CAD build for the part. Positions are in the model's coordinates, mm. Face numbers are marked on the shaded views. A direction names the side the tool comes from. Coordinates: 2 decimals unless noted, no trailing zeros. Write each loop counter-clockwise with the first axis right and the second up, starting at its lowest first coordinate (ties: lowest second). Pieces come first, ordered by that corner, then holes. Notation, with made-up numbers: (-40, 15) -> (-22, 15) arc R24 ccw to (-22, 38) -> close; hole circle Ø5 at (40.5, -30.5). An arc over 180 degrees is marked (long way). Answer as CSV lines item,"result".
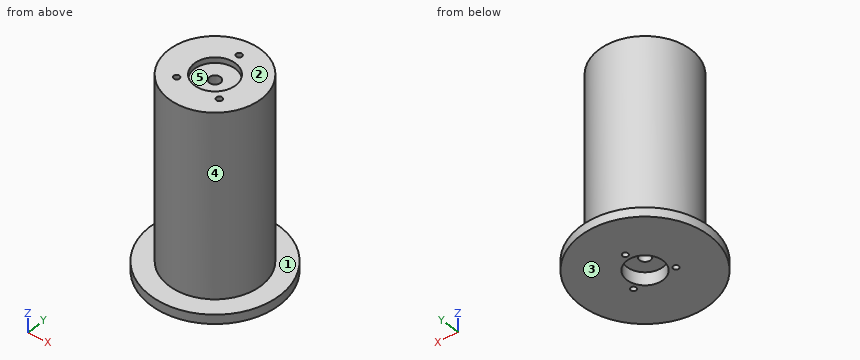
```python
from build123d import *

# Parameters (mm, degrees)
SKETCH_1_R          = 25
EXTRUDE_1_DEPTH     = 100
SKETCH_2_R          = 35
EXTRUDE_2_DEPTH     = 5
SKETCH_4_R          = 9.8
CUT_EXTRUDE_1_DEPTH = 7
SKETCH_5_R          = 3
CUT_EXTRUDE_2_DEPTH = 106
SKETCH_6_R          = 1.5
CUT_EXTRUDE_3_DEPTH = 10
SKETCH_7_R          = 11.15
CUT_EXTRUDE_4_DEPTH = 3
SKETCH_8_R          = 1.55
CUT_EXTRUDE_5_DEPTH = 10


with BuildPart() as part:
    # Эскиз1 → Бобышка-Вытянуть1 (new body)
    with BuildSketch(Plane.XY):
        Circle(SKETCH_1_R)
    extrude(amount=EXTRUDE_1_DEPTH)

    # Эскиз2 → Бобышка-Вытянуть2 (add)
    with BuildSketch(Plane(origin=(0, 0, 0), x_dir=(-1, 0, 0), z_dir=(0, 0, -1))):
        Circle(SKETCH_2_R)
    extrude(amount=EXTRUDE_2_DEPTH)

    # Эскиз4 → Вырез-Вытянуть1 (cut)
    with BuildSketch(Plane(origin=(0, 0, -5), x_dir=(-1, 0, 0), z_dir=(0, 0, -1))):
        Circle(SKETCH_4_R)
    extrude(amount=-CUT_EXTRUDE_1_DEPTH, mode=Mode.SUBTRACT)

    # Эскиз5 → Вырез-Вытянуть2 (cut, through all)
    with BuildSketch(Plane(origin=(0, 0, -5), x_dir=(-1, 0, 0), z_dir=(0, 0, -1))):
        Circle(SKETCH_5_R)
    extrude(amount=-CUT_EXTRUDE_2_DEPTH, mode=Mode.SUBTRACT)

    # Эскиз6 → Вырез-Вытянуть3 (cut)
    with BuildSketch(Plane(origin=(0, 0, -5), x_dir=(-1, 0, 0), z_dir=(0, 0, -1))):
        with Locations((0, 13)):
            Circle(SKETCH_6_R)
        with Locations((11.258330249, -6.5)):
            Circle(SKETCH_6_R)
        with Locations((-11.258330249, -6.5)):
            Circle(SKETCH_6_R)
    extrude(amount=-CUT_EXTRUDE_3_DEPTH, mode=Mode.SUBTRACT)

    # Эскиз7 → Вырез-Вытянуть4 (cut)
    with BuildSketch(Plane.XY.offset(100)):
        Circle(SKETCH_7_R)
    extrude(amount=-CUT_EXTRUDE_4_DEPTH, mode=Mode.SUBTRACT)

    # Эскиз8 → Вырез-Вытянуть5 (cut)
    with BuildSketch(Plane.XY.offset(100)):
        with Locations((0, 16)):
            Circle(SKETCH_8_R)
        with Locations((-11.313708499, -11.313708499)):
            Circle(SKETCH_8_R)
        with Locations((11.313708499, -11.313708499)):
            Circle(SKETCH_8_R)
    extrude(amount=-CUT_EXTRUDE_5_DEPTH, mode=Mode.SUBTRACT)


solid = part.part
```
Item 1: Saw through at D-D on x = 28. Give the cut face in (y, z), and give its area (3 significant figures).
Answer below:
outline,"(-21, -5) -> (21, -5) -> (21, 0) -> (-21, 0) -> close"
area,"210 mm2"
Item 2: Saw through at C-C on y = 13. Give the cut face in (x, z), and give its area (3 significant figures).
Answer below:
outline,"(-32.5, -5) -> (-1.5, -5) -> (-1.5, 5) -> (1.5, 5) -> (1.5, -5) -> (32.5, -5) -> (32.5, 0) -> (21.35, 0) -> (21.35, 100) -> (-21.35, 100) -> (-21.35, 0) -> (-32.5, 0) -> close"
area,"4,570 mm2"
Item 3: Saw through at A-A on x = 0. Give the cut face in (y, z).
Answer below:
outline,"(-35, -5) -> (-9.8, -5) -> (-9.8, 2) -> (-3, 2) -> (-3, 97) -> (-11.15, 97) -> (-11.15, 100) -> (-25, 100) -> (-25, 0) -> (-35, 0) -> close; (3, 2) -> (9.8, 2) -> (9.8, -5) -> (11.5, -5) -> (11.5, 5) -> (14.5, 5) -> (14.5, -5) -> (35, -5) -> (35, 0) -> (25, 0) -> (25, 100) -> (17.55, 100) -> (17.55, 90) -> (14.45, 90) -> (14.45, 100) -> (11.15, 100) -> (11.15, 97) -> (3, 97) -> close"
Item 4: Flat gauge pins, fed straight in: pin 1 (5.5 mm diameter, centred on x = 0, y = 0, fed in from -Z); pin 2 (2 mm diameter, centred on y = 11, z = 18.5, fed in from -X); pin 3 (12 mm diameter, centred on y = 13.5, z = 70, fed in from +X); pin 4 (6 mm diameter, centred on x = 27.5, y = 7.5, fed in from +Z). Where does each tip first touch, or does it go through?
Answer below:
pin 1,"passes through"
pin 2,"stops at x = -22.91"
pin 3,"stops at x = 23.85"
pin 4,"stops at z = 0"
Item 5: Wall check: line 1 (Y direction, x = 0, z = 93); line 2 (Y direction, x = 0, z = 0.5); line 3 (Z direction, x = -20.5, y = -25). Give the ranges that are in metal, low to high. Write a range as from..to.
Answer below:
line 1,"y = -25..-3, 3..14.45, 17.55..25"
line 2,"y = -25..-9.8, 9.8..11.5, 14.5..25"
line 3,"z = -5..0"
Item 6: 3-axis set-ups, long thin cutter, end or side, ignore diameter. For the marked faces 1 and 2: which of +Z, -Z, +X, -X, +Y, -Y reach the whole face in a straight line?
Answer below:
face 1,"+Z"
face 2,"+Z, +X, -X, +Y, -Y"
Item 7: Saw through at B-B on z = 66.5. Give the cut face in (x, y).
Answer below:
outline,"circle Ø50 at (0, 0); hole circle Ø6 at (0, 0)"
Item 8: Two-plate mould, pull along Y, no slides. Class the marked faces 3, 4 and 5: pulls with the +Y half, pulls with the -Y half, needs draft (parallel to the pull), parting line crosses it, or undercut.
Answer below:
face 3,"needs draft"
face 4,"parting line crosses it"
face 5,"undercut"
